The model under review builds one solid part; all positions refer to its coordinate system, in mm. A direction names the side the tool comes from. Round coordinates to 2 decimals unless told otherwise and drop trailing zeros. Write each loop counter-clockwise with the first axis right and the second up, starting at its lowest first coordinate (ties: lowest second). Pieces come first, ordered by that corner, then holes. Notation, with made-up numbers: (6.5, 29.25) - (28.5, 29.25) arc R26 ccw to (28.5, 48.25) - close; hole circle Ø1 at (-23.75, 85.5). An arc over 180 degrees is marked (long way). Use one line per item in the form item = value.
Autodesk Inventor part; units mm, degrees
ref_plane "YZ Plane" through (0, 0, 0) normal (1, 0, 0) x (0, 1, 0)
ref_plane "XZ Plane" through (0, 0, 0) normal (0, 1, 0) x (-1, 0, 0)
ref_plane "XY Plane" through (0, 0, 0) normal (0, 0, 1) x (1, 0, 0)
sketch "Sketch1" plane through (0, 0, 0) normal (0, 1, 0) x (-1, 0, 0)
  line L0 (0, 0) -> (-45.72, 0)
  line L1 (-45.72, 0) -> (-45.72, -21.336)
  line L2 (-45.72, -21.336) -> (0, -21.336)
  line L3 (0, -21.336) -> (0, 0)
  circle A0 centre (-2.54, -2.54) radius 1.5875
  circle A1 centre (-43.18, -18.796) radius 1.5875
  line L4 (-22.86, -21.336) -> (-22.86, 0) construction
  circle A2 centre (-22.86, -1.27) radius 0.127
  circle A3 centre (-20.32, -1.27) radius 0.127
  circle A4 centre (-25.4, -1.27) radius 0.127
  dimension "d0" = 21.336
  dimension "d1" = 45.72
  dimension "d2" = 3.175
  dimension "d3" = 2.54
  dimension "d4" = 2.54
  dimension "d5" = 3.175
  dimension "d6" = 2.54
  dimension "d7" = 2.54
  dimension "d9" = 0.254
  dimension "d10" = 0.254
  dimension "d11" = 0.254
  dimension "d12" = 2.54
  dimension "d13" = 2.54
  dimension "d14" = 1.27
extrude "Extrusion1" add sketch "Sketch1" along normal blind 1.57
sketch "Sketch2" plane through (0, 1.57, 0) normal (0, 1, 0) x (1, 0, 0)
  circle A0 centre (10.16, 10.668) radius 8.128
  line L0 (45.72, 21.336) -> (0, 21.336)
  line L1 (22.86, 21.336) -> (22.86, 0) construction
  line L2 (0, 0) -> (45.72, 0)
  line L3 (0, 21.336) -> (0, 0)
  circle A1 centre (35.56, 10.668) radius 8.128
  dimension "d17" = 10.16
  dimension "d18" = 16.256
  dimension "d19" = 10.668
extrude "Extrusion2" add sketch "Sketch2" along normal blind 13.7
fillet "Fillet1" radius 2.54 1 edges at (2.032, 15.27, -10.668)
fillet "Fillet2" radius 2.54 1 edges at (27.432, 15.27, -10.668)
properties part number "ping"
(1) Add section B-B on y = 5. Write out the cut boundary in (x, z).
Geometry results:
outline = circle Ø16.26 at (10.16, -10.67); circle Ø16.26 at (35.56, -10.67)
(2) Add section C-C on x = 21.5. Write out the cut boundary in (y, z).
Geometry results:
outline = (0, -21.34) - (1.57, -21.34) - (1.57, 0) - (0, 0) - close
(3) Add section A-A on x = 35.56. Write out the cut boundary in (y, z), then the cut area to 3 significant figures.
Geometry results:
outline = (0, -21.34) - (1.57, -21.34) - (1.57, -18.8) - (12.73, -18.8) arc R2.54 ccw to (15.27, -16.26) - (15.27, -5.08) arc R2.54 ccw to (12.73, -2.54) - (1.57, -2.54) - (1.57, 0) - (0, 0) - close
area = 253 mm2
(4) To check wall thickness, follow L1, parallel to Z at x = 20.32, y = 0.45; L2, parallel to Z at x = 2.54, y = 0.7; L3, parallel to Y at x = 17, z = -4.25. State the ranges of each line that lie inside material, in increasing order.
Geometry results:
L1 = -21.34 to -1.4, -1.14 to 0
L2 = -21.34 to -4.13, -0.95 to 0
L3 = 0 to 1.57
(5) Machinability: for faces 1 (the cylindrical face through (27.44, 7.07, -10.31)), 2 (the flat face through (0, 1, -11)), which of the approach directions +Z, -Z, +X, -X, +Y, -Y give a long, thin tool a straight path to every point of the face, cutting with its end or side? Answer none if there is none.
Geometry results:
face_1 = +Y
face_2 = +Z, -Z, -X, +Y, -Y
(6) The part is to be moulded in two halves that separate along Z. For faces 3 (the flat face through (23, 1, 0)), 4 (the cylindrical face through (44.766, 0.774, -18.866)), 5 (the cylindrical face through (8.398, 7.072, -18.603)), 6 (the cylindrical face through (3.8, 0.774, -1.574)), say which applies: +Z half, -Z half, draft (parallel to the pull), parting line (faces both ways), or undercut.
Geometry results:
face_3 = +Z half
face_4 = undercut
face_5 = parting line
face_6 = undercut
(7) Insertion check: P1, Ø5, axis at y = 13.5, z = -5.5, coming from the -X side; P2, Ø4, axis at x = 30, z = -11, coming from the -Y side; P3, Ø4, axis at y = 9.5, z = -13.5, coming from the -X side; P4, Ø5, axis at y = 6, z = -4, coming from the -X side. Each pin has a flat end and moves straight along its axis. Give the tip position at first contact, or say it passes through.
Geometry results:
P1 = 2.51
P2 = 0
P3 = 2.07
P4 = 3.18
